Could you check a few things on this drawing? It's one solid part, dimensions in mm from its lowest x, y, z. A direction names the side the tool comes from. Coordinates: 2 decimals unless noted, no trailing zeros. Write each loop counter-clockwise with the first axis right and the second up, starting at its lowest first coordinate (ties: lowest second). Pieces come first, ordered by that corner, then holes.
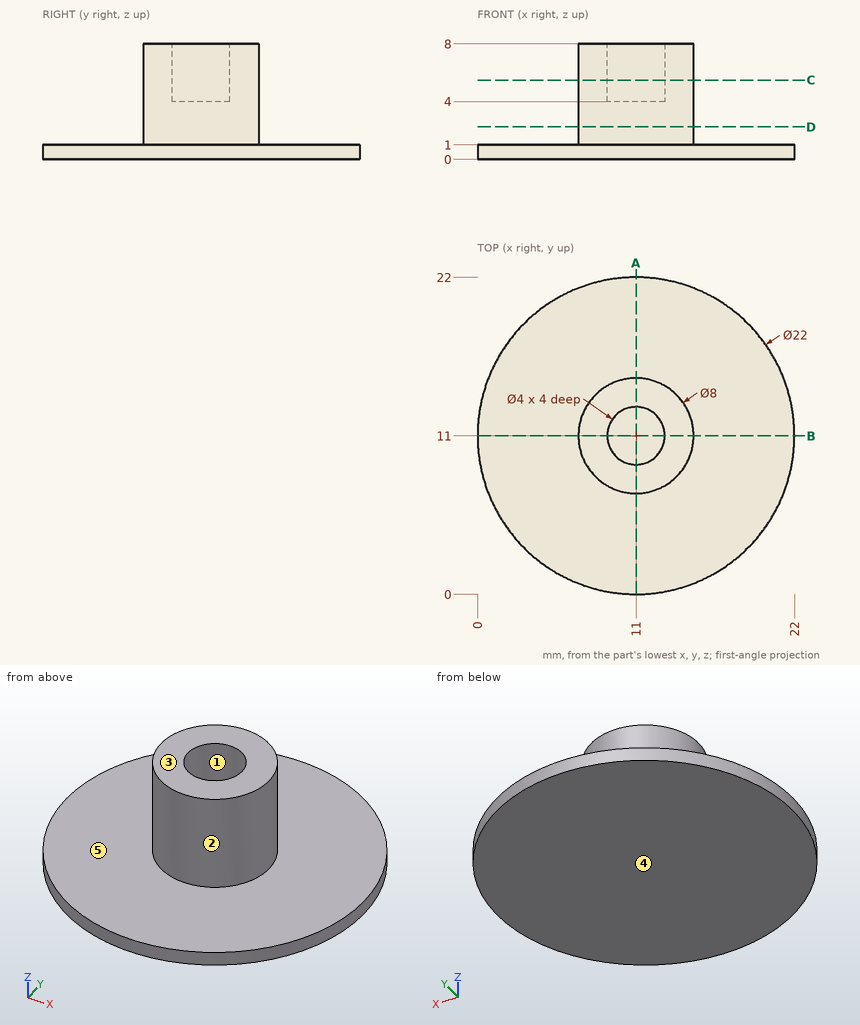
1) Imagine slicing it at A-A on x = 11. Please give me the cut outline in (y, z).
Values follow:
outline: (0, 0) - (22, 0) - (22, 1) - (15, 1) - (15, 8) - (13, 8) - (13, 4) - (9, 4) - (9, 8) - (7, 8) - (7, 1) - (0, 1) - close
2) I need wall thicknesses on probe 1 along Y at (x, z) = (11, 5.7); probe 2 along Z at (x, y) = (18.75, 10.75); probe 3 along X at (y, z) = (11.5, 5.25). Which ranges of each line are inside material? Lowest first, please.
Values follow:
probe 1: y = 7 to 9, 13 to 15
probe 2: z = 0 to 1
probe 3: x = 7.03 to 9.06, 12.94 to 14.97
3) On a 3-axis mill with a long thin cutter (end or side, diameter ignored), from which of +Z, -Z, +X, -X, +Y, -Y can I reach the whole of each face in a straight line? I mean the marked faces 4 and 5. Say none if no direction works.
Values follow:
face 4: -Z, +X, -X, +Y, -Y
face 5: +Z
4) We'd pull the mould along X, two halves only. Please class the marked faces 1, 2 and 3: pulls with the +X half, pulls with the -X half, needs draft (parallel to the pull), parting line crosses it, or undercut.
Values follow:
face 1: undercut
face 2: parting line crosses it
face 3: needs draft
5) Imagine slicing it at C-C on z = 5.5. Please give me the cut outline in (x, y).
Values follow:
outline: circle Ø8 at (11, 11); hole circle Ø4 at (11, 11)
6) Will these pins go through, and if not, where does the flat tip stop? pin 1 (3.5 mm diameter, centred on x = 11, y = 11, fed in from +Z); pin 2 (3 mm diameter, centred on x = 14.5, y = 6.5, fed in from +Z); pin 3 (3 mm diameter, centred on x = 17.5, z = 4, fed in from +Y); pin 4 (4 mm diameter, centred on x = 10.5, z = 6, fed in from -Y).
Values follow:
pin 1: stops at z = 4
pin 2: stops at z = 1
pin 3: passes through
pin 4: stops at y = 7
7) Imagine slicing it at D-D on z = 2.25. Please give me the cut outline in (x, y), then the cut area to 3 significant figures.
Values follow:
outline: circle Ø8 at (11, 11)
area: 50.3 mm2
